from build123d import *

# Parameters (mm, degrees)
F1_DEPTH = 12.7
F2_R     = 46.63803
F3_DEPTH = 25.4


with BuildPart() as f1:
    # F0 (on Front) → F1 (new body)
    with BuildSketch(Plane.XZ):
        with BuildLine():
            ThreePointArc((-63.765545, 12.165316), (-64.250755, 9.267153), (-64.604312, 6.35))
            Line((-64.604312, 6.35), (-75.607494, 6.35))
            Line((-75.607494, 6.35), (-75.607494, 0))
            Line((-75.607494, 0), (-75.607494, -6.35))
            Line((-75.607494, -6.35), (-64.604312, -6.35))
            ThreePointArc((-64.604312, -6.35), (-64.250755, -9.267153), (-63.765545, -12.165316))
            Line((-63.765545, -12.165316), (-74.686304, -15.897153))
            Line((-74.686304, -15.897153), (-70.579622, -27.914854))
            Line((-70.579622, -27.914854), (-60.172292, -24.358467))
            ThreePointArc((-60.172292, -24.358467), (-58.750975, -27.610913), (-57.154014, -30.780811))
            Line((-57.154014, -30.780811), (-66.276509, -36.902763))
            Line((-66.276509, -36.902763), (-59.199606, -47.448258))
            Line((-59.199606, -47.448258), (-50.067208, -41.31966))
            ThreePointArc((-50.067208, -41.31966), (-47.767053, -43.958483), (-45.327995, -46.469479))
            Line((-45.327995, -46.469479), (-52.3023, -54.973564))
            Line((-52.3023, -54.973564), (-42.48234, -63.027035))
            Line((-42.48234, -63.027035), (-35.412164, -54.40605))
            ThreePointArc((-35.412164, -54.40605), (-30.761411, -57.164458), (-25.897226, -59.526241))
            Line((-25.897226, -59.526241), (-29.681084, -69.853042))
            Line((-29.681084, -69.853042), (-17.756371, -74.222393))
            Line((-17.756371, -74.222393), (-13.802402, -63.431328))
            ThreePointArc((-13.802402, -63.431328), (-10.093255, -64.126171), (-6.35, -64.604312))
            Line((-6.35, -64.604312), (-6.35, -75.913835))
            Line((-6.35, -75.913835), (0, -75.913835))
            Line((0, -75.913835), (6.35, -75.913835))
            Line((6.35, -75.913835), (6.35, -64.604312))
            ThreePointArc((6.35, -64.604312), (10.093255, -64.126171), (13.802402, -63.431328))
            Line((13.802402, -63.431328), (17.756371, -74.222393))
            Line((17.756371, -74.222393), (29.681084, -69.853042))
            Line((29.681084, -69.853042), (25.897226, -59.526241))
            ThreePointArc((25.897226, -59.526241), (30.761411, -57.164458), (35.412164, -54.40605))
            Line((35.412164, -54.40605), (42.48234, -63.027035))
            Line((42.48234, -63.027035), (52.3023, -54.973564))
            Line((52.3023, -54.973564), (45.327995, -46.469479))
            ThreePointArc((45.327995, -46.469479), (47.767053, -43.958483), (50.067208, -41.31966))
            Line((50.067208, -41.31966), (59.199606, -47.448258))
            Line((59.199606, -47.448258), (66.276509, -36.902763))
            Line((66.276509, -36.902763), (57.154014, -30.780811))
            ThreePointArc((57.154014, -30.780811), (58.750975, -27.610913), (60.172292, -24.358467))
            Line((60.172292, -24.358467), (70.579622, -27.914854))
            Line((70.579622, -27.914854), (74.686304, -15.897153))
            Line((74.686304, -15.897153), (63.765545, -12.165316))
            ThreePointArc((63.765545, -12.165316), (64.250755, -9.267153), (64.604312, -6.35))
            Line((64.604312, -6.35), (75.607494, -6.35))
            Line((75.607494, -6.35), (75.607494, 0))
            Line((75.607494, 0), (75.607494, 6.35))
            Line((75.607494, 6.35), (64.604312, 6.35))
            ThreePointArc((64.604312, 6.35), (64.250755, 9.267153), (63.765545, 12.165316))
            Line((63.765545, 12.165316), (74.686304, 15.897153))
            Line((74.686304, 15.897153), (70.579622, 27.914854))
            Line((70.579622, 27.914854), (60.172292, 24.358467))
            ThreePointArc((60.172292, 24.358467), (58.750975, 27.610913), (57.154014, 30.780811))
            Line((57.154014, 30.780811), (66.276509, 36.902763))
            Line((66.276509, 36.902763), (59.199606, 47.448258))
            Line((59.199606, 47.448258), (50.067208, 41.31966))
            ThreePointArc((50.067208, 41.31966), (47.767053, 43.958483), (45.327995, 46.469479))
            Line((45.327995, 46.469479), (52.3023, 54.973564))
            Line((52.3023, 54.973564), (42.48234, 63.027035))
            Line((42.48234, 63.027035), (35.412164, 54.40605))
            ThreePointArc((35.412164, 54.40605), (30.761411, 57.164458), (25.897226, 59.526241))
            Line((25.897226, 59.526241), (29.681084, 69.853042))
            Line((29.681084, 69.853042), (17.756371, 74.222393))
            Line((17.756371, 74.222393), (13.802402, 63.431328))
            ThreePointArc((13.802402, 63.431328), (10.093255, 64.126171), (6.35, 64.604312))
            Line((6.35, 64.604312), (6.35, 75.913835))
            Line((6.35, 75.913835), (0, 75.913835))
            Line((0, 75.913835), (-6.35, 75.913835))
            Line((-6.35, 75.913835), (-6.35, 64.604312))
            ThreePointArc((-6.35, 64.604312), (-10.093255, 64.126171), (-13.802402, 63.431328))
            Line((-13.802402, 63.431328), (-17.756371, 74.222393))
            Line((-17.756371, 74.222393), (-29.681084, 69.853042))
            Line((-29.681084, 69.853042), (-25.897226, 59.526241))
            ThreePointArc((-25.897226, 59.526241), (-30.761411, 57.164458), (-35.412164, 54.40605))
            Line((-35.412164, 54.40605), (-42.48234, 63.027035))
            Line((-42.48234, 63.027035), (-52.3023, 54.973564))
            Line((-52.3023, 54.973564), (-45.327995, 46.469479))
            ThreePointArc((-45.327995, 46.469479), (-47.767053, 43.958483), (-50.067208, 41.31966))
            Line((-50.067208, 41.31966), (-59.199606, 47.448258))
            Line((-59.199606, 47.448258), (-66.276509, 36.902763))
            Line((-66.276509, 36.902763), (-57.154014, 30.780811))
            ThreePointArc((-57.154014, 30.780811), (-58.750975, 27.610913), (-60.172292, 24.358467))
            Line((-60.172292, 24.358467), (-70.579622, 27.914854))
            Line((-70.579622, 27.914854), (-74.686304, 15.897153))
            Line((-74.686304, 15.897153), (-63.765545, 12.165316))
        make_face()
    extrude(amount=F1_DEPTH)

    # F2 (on face) → F3 (cut)
    with BuildSketch(Plane.XZ.offset(12.7)):
        Circle(F2_R)
    extrude(amount=-F3_DEPTH, mode=Mode.SUBTRACT)


solid = f1.part
The model under review builds one solid part; all positions refer to its coordinate system, in mm. A direction names the side the tool comes from. Give positions to 0.01 mm unless a question says otherwise; leave off trailing zeros. Write each loop counter-clockwise with the first axis right and the second up, starting at its lowest first coordinate (ties: lowest second). Pieces come first, ordered by that corner, then holes.
1. For P1, Ø6, axis at y = -2, z = 51, coming from the +X side; P2, Ø5.5, axis at x = -70, y = -9, coming from the -Z side; P3, Ø3.5, axis at y = -3.5, z = -70.5, coming from the +X side, all flat-tipped, find the tip position at first contact; note any pin that passes through.
2. Add section B-B, the plane x = 0. Write out the cut boundary in (y, z).
3. Draft analysis for pull direction Z (two halves, no side actions). For faces 6 (the flat face through (-75.607, -6, 0)), 7 (the flat face through (-23.8, -6.26, -72.01)), 8 (the cylindrical face through (-10.041, -6.261, 64.134)), 9 (the cylindrical face through (-58.77, -6.26, -27.57)), state which applies: +Z half, -Z half, draft (parallel to the pull), parting line (faces both ways), or undercut.
4. Tool access review of faces 1 (the flat face through (38.9, -6.26, -58.66)), 2 (the cylindrical face through (-30.828, -6.261, -57.129)), 3 (the flat face through (-61.65, -6.26, -33.8)), 4 (the flat face through (6.35, -6, 70)), 5 (the flat face through (61.8, -6.3, -33.9)): name each direction out of +Z, -Z, +X, -X, +Y, -Y from which nothing blocks a thin tool from reaching the whole face with its end or side.
5. Wall thickness on L1, parallel to Z at x = 60.5, y = -3.5; L2, parallel to Z at x = 48, y = -11.25; L3, parallel to Z at x = 0, y = -8.5: over which ranges is each line inside the solid? List them lowest first.
6. Add section D-D, the plane z = -57. Write out the cut boundary in (x, y), plus the area to 3 significant figures.
7. Add section A-A, the plane z = 0. Write out the cut boundary in (x, y).
8. Add section C-C, the plane z = 43.5. Write out the cut boundary in (x, y).
Worked answers:
1. P1: stops at x = 51.5
1. P2: stops at z = -27.91
1. P3: stops at x = 29.68
2. outline: (-12.7, -75.91) - (0, -75.91) - (0, -46.64) - (-12.7, -46.64) - close; (-12.7, 46.64) - (0, 46.64) - (0, 75.91) - (-12.7, 75.91) - close
3. face 6: draft
3. face 7: -Z half
3. face 8: +Z half
3. face 9: undercut
4. face 1: -Z, +Y, -Y
4. face 2: +Y, -Y
4. face 3: -X, +Y, -Y
4. face 4: +Z, +Y, -Y
4. face 5: +X, +Y, -Y
5. L1: z = -45.51 to -33.03, -24.47 to 24.47, 33.03 to 45.51
5. L2: z = -58.5 to -49.73, -43.7 to 43.7, 49.73 to 58.5
5. L3: z = -75.91 to -46.64, 46.64 to 75.91
6. outline: (-49.83, -12.7) - (-37.54, -12.7) - (-37.54, 0) - (-49.83, 0) - close; (-31.07, -12.7) - (31.07, -12.7) - (31.07, 0) - (-31.07, 0) - close; (37.54, -12.7) - (49.83, -12.7) - (49.83, 0) - (37.54, 0) - close
6. area: 1,100 mm2
7. outline: (-75.61, -12.7) - (-46.64, -12.7) - (-46.64, 0) - (-75.61, 0) - close; (46.64, -12.7) - (75.61, -12.7) - (75.61, 0) - (46.64, 0) - close
8. outline: (-61.85, -12.7) - (-53.32, -12.7) - (-53.32, 0) - (-61.85, 0) - close; (-48.18, -12.7) - (-16.82, -12.7) - (-16.82, 0) - (-48.18, 0) - close; (16.82, -12.7) - (48.18, -12.7) - (48.18, 0) - (16.82, 0) - close; (53.32, -12.7) - (61.85, -12.7) - (61.85, 0) - (53.32, 0) - close
